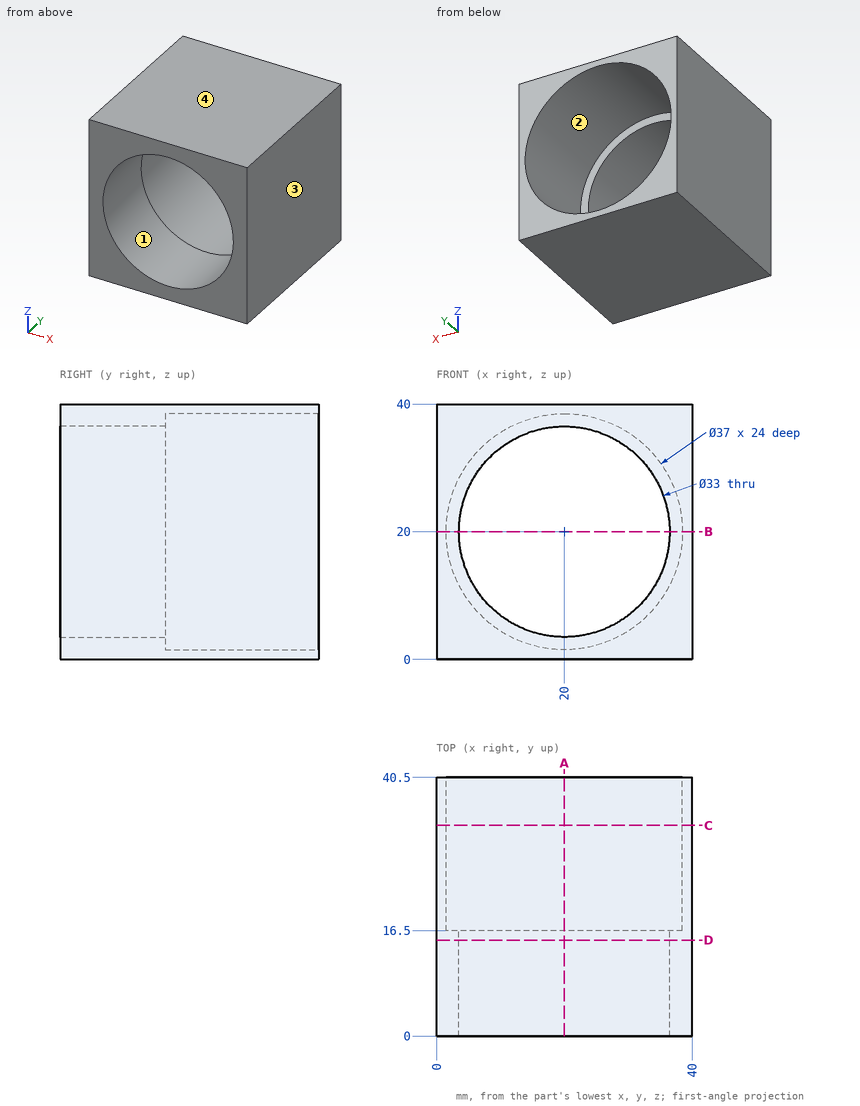
Input: dimensioned drawing with shaded views. Units: mm. Origin: part minimum x, y, z. Coordinates: 2 decimals unless noted, no trailing zeros. Write each loop counter-clockwise with the first axis right and the second up, starting at its lowest first coordinate (ties: lowest second). Pieces come first, ordered by that corner, then holes. Notation, with made-up numbers: (69, -1) -> (95, -1) arc R24 cw to (95, 18) -> close; hole circle Ø11 at (69, 73). An arc over 180 degrees is marked (long way). Return JSON: item names as keys, results as strings. Group by question number.
1) Section query C-C, the plane y = 33. Return loops of the section in (x, z), plus the area to 3 significant figures.
2) Section query D-D, the plane y = 15. Return loops of the section in (x, z).
3) Section query B-B, the plane z = 20. Return loops of the section in (x, y).
4) Mould query, pull axis X, two halves, no side actions, for the marked faces 1, 2, 3 and 4. Classes: +X half, -X half, draft (parallel to the pull), parting line (faces both ways), or undercut.
5) Contact query for a flat-ended pin moving along its axis: P1, Ø2, axis at x = 15, z = 33, coming from the -Y side. Output: stop coordinate, or through.
6) Section query A-A, the plane x = 20. Return loops of the section in (y, z).
7) Ray query, line 1 along X through (y, z) = (33.25, 20); line 2 along Y through (x, z) = (3, 22.5); line 3 along Z through (x, y) = (9.5, 28.5). Return the intervals inside material, ascending.
From the geometry:
{
 "1": {"outline": "(0, 0) -> (40, 0) -> (40, 40) -> (0, 40) -> close; hole circle Ø37 at (20, 20)", "area": "525 mm²"},
 "2": {"outline": "(0, 0) -> (40, 0) -> (40, 40) -> (0, 40) -> close; hole circle Ø33 at (20, 20)"},
 "3": {"outline": "(0, 0) -> (3.5, 0) -> (3.5, 16.5) -> (1.5, 16.5) -> (1.5, 40.5) -> (0, 40.5) -> close; (36.5, 0) -> (40, 0) -> (40, 40.5) -> (38.5, 40.5) -> (38.5, 16.5) -> (36.5, 16.5) -> close"},
 "4": {"face 1": "undercut", "face 2": "undercut", "face 3": "+X half", "face 4": "draft"},
 "5": {"P1": "through"},
 "6": {"outline": "(0, 0) -> (40.5, 0) -> (40.5, 1.5) -> (16.5, 1.5) -> (16.5, 3.5) -> (0, 3.5) -> close; (0, 36.5) -> (16.5, 36.5) -> (16.5, 38.5) -> (40.5, 38.5) -> (40.5, 40) -> (0, 40) -> close"},
 "7": {"line 1": "0 to 1.5, 38.5 to 40", "line 2": "0 to 16.5", "line 3": "0 to 4.77, 35.23 to 40"}
}
